```python
from build123d import *

# Parameters (mm, degrees)
SKETCH2_W           = 50.5
SKETCH2_H           = 40
SKETCH2_W_2         = 42.5
SKETCH2_H_2         = 34
BOSS_EXTRUDE1_DEPTH = 45
CUT_EXTRUDE1_REACH  = 72.825
SKETCH3_W           = 26
SKETCH3_H           = 27.5
CUT_EXTRUDE2_REACH  = 67.288
SKETCH4_R           = 11.5
SKETCH4_R_2         = 1.6
CUT_EXTRUDE3_REACH  = 67.288
SKETCH5_R           = 3
CUT_EXTRUDE4_REACH  = 67.288
SKETCH6_R           = 2.75
SKETCH7_R           = 2.75
CUT_EXTRUDE5_DEPTH  = 71.825489762
SKETCH8_W           = 8
SKETCH8_H           = 25
BOSS_EXTRUDE2_DEPTH = 4
SKETCH9_R           = 2.25
CUT_EXTRUDE6_DEPTH  = 4
CHAMFER1_SIZE       = 0.75


with BuildPart() as part:
    # Sketch2 → Boss-Extrude1 (new body)
    with BuildSketch(Plane(origin=(0, 0, 0), x_dir=(1, 0, 0), z_dir=(0, 1, 0))):
        with Locations((0, -1)):
            Rectangle(SKETCH2_W, SKETCH2_H)
        Rectangle(SKETCH2_W_2, SKETCH2_H_2, mode=Mode.SUBTRACT)
    extrude(amount=BOSS_EXTRUDE1_DEPTH)

    # Sketch3 → Cut-Extrude1 (cut, up to next)
    with BuildSketch(Plane(origin=(25.25, 0, 0), x_dir=(0, 0, -1), z_dir=(1, 0, 0)), mode=Mode.PRIVATE) as cut_extrude1_sk1:
        with Locations((-1, 31.25)):
            Rectangle(SKETCH3_W, SKETCH3_H)
    cut_extrude1_tool1 = extrude(cut_extrude1_sk1.sketch, amount=-CUT_EXTRUDE1_REACH, mode=Mode.PRIVATE) & part.part
    add(cut_extrude1_tool1.solids().sort_by_distance((25.25, 31.25, 1))[0], mode=Mode.SUBTRACT)

    # Sketch4 → Cut-Extrude2 (cut, up to next)
    with BuildSketch(Plane(origin=(0, 0, -19), x_dir=(-1, 0, 0), z_dir=(0, 0, -1)), mode=Mode.PRIVATE) as cut_extrude2_sk1:
        with Locations((0, 21)):
            Circle(SKETCH4_R)
    cut_extrude2_tool1 = extrude(cut_extrude2_sk1.sketch, amount=-CUT_EXTRUDE2_REACH, mode=Mode.PRIVATE) & part.part
    # Sketch4 → Cut-Extrude2 (cut, up to next)
    with BuildSketch(Plane(origin=(0, 0, -19), x_dir=(-1, 0, 0), z_dir=(0, 0, -1)), mode=Mode.PRIVATE) as cut_extrude2_sk2:
        with Locations((-15.5, 5.5)):
            Circle(SKETCH4_R_2)
    cut_extrude2_tool2 = extrude(cut_extrude2_sk2.sketch, amount=-CUT_EXTRUDE2_REACH, mode=Mode.PRIVATE) & part.part
    # Sketch4 → Cut-Extrude2 (cut, up to next)
    with BuildSketch(Plane(origin=(0, 0, -19), x_dir=(-1, 0, 0), z_dir=(0, 0, -1)), mode=Mode.PRIVATE) as cut_extrude2_sk3:
        with Locations((15.5, 5.5)):
            Circle(SKETCH4_R_2)
    cut_extrude2_tool3 = extrude(cut_extrude2_sk3.sketch, amount=-CUT_EXTRUDE2_REACH, mode=Mode.PRIVATE) & part.part
    # Sketch4 → Cut-Extrude2 (cut, up to next)
    with BuildSketch(Plane(origin=(0, 0, -19), x_dir=(-1, 0, 0), z_dir=(0, 0, -1)), mode=Mode.PRIVATE) as cut_extrude2_sk4:
        with Locations((15.5, 36.5)):
            Circle(SKETCH4_R_2)
    cut_extrude2_tool4 = extrude(cut_extrude2_sk4.sketch, amount=-CUT_EXTRUDE2_REACH, mode=Mode.PRIVATE) & part.part
    add(cut_extrude2_tool1.solids().sort_by_distance((0, 21, -19))[0], mode=Mode.SUBTRACT)
    add(cut_extrude2_tool2.solids().sort_by_distance((15.5, 5.5, -19))[0], mode=Mode.SUBTRACT)
    add(cut_extrude2_tool3.solids().sort_by_distance((-15.5, 5.5, -19))[0], mode=Mode.SUBTRACT)
    add(cut_extrude2_tool4.solids().sort_by_distance((-15.5, 36.5, -19))[0], mode=Mode.SUBTRACT)

    # Sketch5 → Cut-Extrude3 (cut, up to next)
    with BuildSketch(Plane.XY.offset(21), mode=Mode.PRIVATE) as cut_extrude3_sk1:
        with Locations((-15.5, 36.5)):
            Circle(SKETCH5_R)
    cut_extrude3_tool1 = extrude(cut_extrude3_sk1.sketch, amount=-CUT_EXTRUDE3_REACH, mode=Mode.PRIVATE) & part.part
    # Sketch5 → Cut-Extrude3 (cut, up to next)
    with BuildSketch(Plane.XY.offset(21), mode=Mode.PRIVATE) as cut_extrude3_sk2:
        with Locations((-15.5, 5.5)):
            Circle(SKETCH5_R)
    cut_extrude3_tool2 = extrude(cut_extrude3_sk2.sketch, amount=-CUT_EXTRUDE3_REACH, mode=Mode.PRIVATE) & part.part
    # Sketch5 → Cut-Extrude3 (cut, up to next)
    with BuildSketch(Plane.XY.offset(21), mode=Mode.PRIVATE) as cut_extrude3_sk3:
        with Locations((15.5, 5.5)):
            Circle(SKETCH5_R)
    cut_extrude3_tool3 = extrude(cut_extrude3_sk3.sketch, amount=-CUT_EXTRUDE3_REACH, mode=Mode.PRIVATE) & part.part
    add(cut_extrude3_tool1.solids().sort_by_distance((-15.5, 36.5, 21))[0], mode=Mode.SUBTRACT)
    add(cut_extrude3_tool2.solids().sort_by_distance((-15.5, 5.5, 21))[0], mode=Mode.SUBTRACT)
    add(cut_extrude3_tool3.solids().sort_by_distance((15.5, 5.5, 21))[0], mode=Mode.SUBTRACT)

    # Sketch6 → Cut-Extrude4 (cut, up to next)
    with BuildSketch(Plane.XY.offset(21), mode=Mode.PRIVATE) as cut_extrude4_sk1:
        with Locations((-15.5, 16.365063509)):
            Circle(SKETCH6_R)
    cut_extrude4_tool1 = extrude(cut_extrude4_sk1.sketch, amount=-CUT_EXTRUDE4_REACH, mode=Mode.PRIVATE) & part.part
    # Sketch6 → Cut-Extrude4 (cut, up to next)
    with BuildSketch(Plane.XY.offset(21), mode=Mode.PRIVATE) as cut_extrude4_sk2:
        with Locations((0, 5.5)):
            Circle(SKETCH6_R)
    cut_extrude4_tool2 = extrude(cut_extrude4_sk2.sketch, amount=-CUT_EXTRUDE4_REACH, mode=Mode.PRIVATE) & part.part
    # Sketch6 → Cut-Extrude4 (cut, up to next)
    with BuildSketch(Plane.XY.offset(21), mode=Mode.PRIVATE) as cut_extrude4_sk3:
        with Locations((15.5, 16.365063509)):
            Circle(SKETCH6_R)
    cut_extrude4_tool3 = extrude(cut_extrude4_sk3.sketch, amount=-CUT_EXTRUDE4_REACH, mode=Mode.PRIVATE) & part.part
    add(cut_extrude4_tool1.solids().sort_by_distance((-15.5, 16.365064, 21))[0], mode=Mode.SUBTRACT)
    add(cut_extrude4_tool2.solids().sort_by_distance((0, 5.5, 21))[0], mode=Mode.SUBTRACT)
    add(cut_extrude4_tool3.solids().sort_by_distance((15.5, 16.365064, 21))[0], mode=Mode.SUBTRACT)

    # Sketch7 → Cut-Extrude5 (cut, through all)
    with BuildSketch(Plane(origin=(25.25, 0, 0), x_dir=(0, 0, -1), z_dir=(1, 0, 0))):
        with Locations((-11, 13.440603491)):
            Circle(SKETCH7_R)
        with Locations((9, 13.440603491)):
            Circle(SKETCH7_R)
    extrude(amount=-CUT_EXTRUDE5_DEPTH, mode=Mode.SUBTRACT)

    # Sketch8 → Boss-Extrude2 (add)
    with BuildSketch(Plane.XZ):
        Polygon((19, 1), (17.25, 11), (17.25, 21), (25.25, 21), (25.25, 1), align=None)
        with Locations((-21.25, 8.5)):
            Rectangle(SKETCH8_W, SKETCH8_H)
    extrude(amount=BOSS_EXTRUDE2_DEPTH)

    # Sketch9 → Cut-Extrude6 (cut)
    with BuildSketch(Plane.XZ.offset(4)):
        with Locations(Location((-21.25, 13, 0), (0, 0, 270))):
            Circle(SKETCH9_R)
        with Locations(Location((-21.25, 0.5, 0), (0, 0, 270))):
            Circle(SKETCH9_R)
        with Locations(Location((21.25, 6, 0), (0, 0, 270))):
            Circle(SKETCH9_R)
        with Locations(Location((21.25, 16, 0), (0, 0, 270))):
            Circle(SKETCH9_R)
    extrude(amount=-CUT_EXTRUDE6_DEPTH, mode=Mode.SUBTRACT)

    # Chamfer1
    chamfer1_edges = [part.edges().sort_by_distance(p)[0] for p in [
        (21.25, -4, 18.25),
        (21.25, -4, 8.25),
        (-21.25, -4, 2.75),
        (-21.25, -4, 15.25),
        (-18.25, 16.365063509, 21),
        (-2.75, 5.5, 21),
        (12.75, 16.365063509, 21),
        (-25.25, 13.440603491, 13.75),
        (25.25, 13.440603491, 13.75),
        (-25.25, 13.440603491, -6.25),
        (25.25, 13.440603491, -6.25),
    ]]
    chamfer(chamfer1_edges, length=CHAMFER1_SIZE)


solid = part.part
```
Could you check a few things on this model? Use its own coordinates, in mm. A direction names the side the tool comes from. Coordinates: 2 decimals unless noted, no trailing zeros. Write each loop counter-clockwise with the first axis right and the second up, starting at its lowest first coordinate (ties: lowest second). Pieces come first, ordered by that corner, then holes. Notation, with made-up numbers: (87.25, 25) -> (126.25, 25) arc R17 cw to (126.25, 56) -> close; hole circle Ø5 at (-19, -2). An arc over 180 degrees is marked (long way). Write item = value, one per line. Start each with the question number.
(1) I want a section at B-B (y = 5.5). Give the number of separate pieces and of enclosed holes in the cut face, plus the area to 3 significant figures.
(2) I want a section at C-C (x = 15.5). Please give me the cut outline in (y, z).
(3) I want a section at D-D (z = 6). Please give me the cut outline in (x, y) (3 decimals), plus the area to 3 significant figures.
(4) I want a section at A-A (x = 0). Please give me the cut outline in (y, z), plus the area to 3 significant figures.
(5) Will these pins go through, and if not, where does the flat tip stop? pin 1 (10 mm diameter, centred on x = 6, z = 10, fed in from -Y); pin 2 (5 mm diameter, centred on x = -15.5, y = 36.5, fed in from +Z); pin 3 (2.5 mm diameter, centred on x = 22.5, z = 6.5, fed in from -Y); pin 4 (1.2 mm diameter, centred on x = -19.5, z = 4.5, fed in from +Y).
(6) I need wall thicknesses on line 1 (Y direction, x = -15.5, z = -18.1); line 2 (X direction, y = 9.5, z = 0.5); line 3 (Z direction, x = 16, y = 28.5). Which ranges of each line are inside material? Lowest first, please. Write a range as [from, to].
(7) We'd pull the mould along Z, two halves only. Please class faces 4 (the face through (-21.25, 22, 0)), 5 (the face through (-22, 0, 1)), 6 (the face through (-17.71, 38.53, 19.03)), 7 (the face through (-12, 22, -19)): released by +Z, released by -Z, zero draft, split by the parting line, or undercut.
(8) Which directions (+Z, -Z, +X, -X, +Y, -Y) give clear straight access to the entire face, cutting with the end or side of a thin tool? Please do faces 1 (the face through (-23.446, -1.648, 0.988)), 2 (the face through (23, 31, 14)), 3 (the face through (0, 0, 19)).
Result set:
q1.separate_pieces = 5
q1.enclosed_holes = 0
q1.area = 492 mm2
q2.outline = (0, -19) -> (3.9, -19) -> (3.9, -17) -> (0, -17) -> close; (0, 17) -> (2.5, 17) -> (2.5, 21) -> (0, 21) -> close; (7.1, -19) -> (45, -19) -> (45, -17) -> (7.1, -17) -> close; (8.5, 17) -> (13.62, 17) -> (13.62, 20.25) -> (12.87, 21) -> (8.5, 21) -> close; (19.12, 17) -> (45, 17) -> (45, 21) -> (19.87, 21) -> (19.12, 20.25) -> close
q3.outline = (-25.25, -4) -> (-17.25, -4) -> (-17.25, 0) -> (-21.25, 0) -> (-21.25, 45) -> (-25.25, 45) -> close; (18.125, -4) -> (18.25, -4) -> (19, -3.25) -> (19, 0) -> (18.125, 0) -> close; (21.25, 0) -> (23.5, 0) -> (23.5, -3.25) -> (24.25, -4) -> (25.25, -4) -> (25.25, 17.5) -> (21.25, 17.5) -> close
q3.area = 292 mm2
q4.outline = (0, -19) -> (9.5, -19) -> (9.5, -17) -> (0, -17) -> close; (0, 17) -> (2.75, 17) -> (2.75, 20.25) -> (2, 21) -> (0, 21) -> close; (8.25, 17) -> (45, 17) -> (45, 21) -> (9, 21) -> (8.25, 20.25) -> close; (32.5, -19) -> (45, -19) -> (45, -17) -> (32.5, -17) -> close
q4.area = 201 mm2
q5.pin_1 = through
q5.pin_2 = -17
q5.pin_3 = -3.6
q5.pin_4 = 0
q6.line_1 = [0, 3.9], [7.1, 34.9], [38.1, 45]
q6.line_2 = [-25.25, -21.25], [21.25, 25.25]
q6.line_3 = [-19, -17], [17, 21]
q7.face_4 = undercut
q7.face_5 = undercut
q7.face_6 = zero draft
q7.face_7 = released by -Z
q8.face_1 = -Y
q8.face_2 = +X, +Y
q8.face_3 = +Z, -Z, -Y
